The model under review builds one solid part; all positions refer to its coordinate system, in mm. A direction names the side the tool comes from. Coordinates: 2 decimals unless noted, no trailing zeros. Write each loop counter-clockwise with the first axis right and the second up, starting at its lowest first coordinate (ties: lowest second). Pieces come first, ordered by that corner, then holes. Notation, with made-up numbers: (-38.75, 80) - (-11.75, 80) arc R19 cw to (-11.75, 93) - close; hole circle Ø3 at (-34.75, 2.25). An arc over 180 degrees is marked (long way). Put each result on its own line as item: value. Start each with the question number.
Item 1: Consider section D-D on y = -10.5. Give the boundary of the cut face in (x, z), then the cut area to 3 significant figures.
Item 2: Consider section B-B on z = -35. Give the boundary of the cut face in (x, y).
Item 3: Consider section A-A on x = -32.5. Give the boundary of the cut face in (y, z).
Item 4: Consider section C-C on y = 0. State how many separate pieces and enclosed holes the cut face has, then the cut area to 3 significant figures.
Item 5: For pin 1 (6 mm diameter, centred on x = -101.5, y = -4.5, fed in from +Z); pin 2 (15.5 mm diameter, centred on y = -4, z = -22.5, fed in from +X); pin 3 (5 mm diameter, centred on x = -105, y = 0, fed in from -Z); pin 4 (2 mm diameter, centred on x = 0, y = -12, fed in from -Z), all flat-tipped, find the tip position at first contact; note any pin that passes through.
Item 6: Mouldability with a two-part tool opening along X and no side actions: class faces 4 (the face through (-93, 0, -23)), 5 (the face through (95, 0, -23)), 6 (the face through (-95, 0, -22)), 7 (the face through (-107, -4, -38)) as pulls with the +X half, pulls with the -X half, needs draft (parallel to the pull), parting line crosses it, or undercut.
Item 7: To check wall thickness, follow L1, parallel to X at y = 13, z = -18.5; L2, parallel to Z at x = -102.5, y = 13.5; L3, parallel to Y at x = 32, z = -6. State the ranges of each line that lie inside material, in increasing order. Write a range as [from, to].
Item 8: Machinability: for faces 1 (the face through (-1, 0, -7)), 2 (the face through (107, -4, -38)), 3 (the face through (-107, -4, -40)), which of the approach directions +Z, -Z, +X, -X, +Y, -Y give a long, thin tool a straight path to every point of the face, cutting with its end or side? Answer none if there is none.
```python
from build123d import *

# Parameters (mm, degrees)
F1_DEPTH = 17.5
F2_R     = 4
F3_DEPTH = 25
F4_R     = 4.4
F5_DEPTH = 25
F6_R     = 2


# Not quite as in the source:
# - a feature names something its author has since deleted; it is built from what else it names


with BuildPart() as f1:
    # F0 (on Front) → F1 (new body, symmetric)
    with BuildSketch(Plane.XZ):
        Polygon((95, -38), (95, -5), (-95, -5), (-95, -38), (-115, -38), (-115, -40), (-93, -40), (-93, -7), (93, -7), (93, -40), (115, -40), (115, -38), align=None)
    extrude(amount=F1_DEPTH, both=True)

    # F2 (on face) → F3 (cut)
    with BuildSketch(Plane.XY.offset(-38)):
        with Locations((-105, 0)):
            Circle(F2_R)
        with Locations((105, 0)):
            Circle(F2_R)
    extrude(amount=-F3_DEPTH, mode=Mode.SUBTRACT)

    # F4 (on face) → F5 (cut)
    with BuildSketch(Plane.XY.offset(-5)):
        with Locations((-32.5, 0)):
            Circle(F4_R)
        with Locations((32.5, 0)):
            Circle(F4_R)
    extrude(amount=-F5_DEPTH, mode=Mode.SUBTRACT)

    # F6
    f6_edges = [f1.edges().sort_by_distance(p)[0] for p in [
        (95, 0, -5),
        (-95, 0, -5),
        (-93, 0, -40),
        (93, 0, -40),
    ]]
    fillet(f6_edges, radius=F6_R)


solid = f1.part
```
Report:
1. outline: (-115, -40) - (-95, -40) arc R2 ccw to (-93, -38) - (-93, -7) - (93, -7) - (93, -38) arc R2 ccw to (95, -40) - (115, -40) - (115, -38) - (95, -38) - (95, -7) arc R2 ccw to (93, -5) - (-93, -5) arc R2 ccw to (-95, -7) - (-95, -38) - (-115, -38) - close
1. area: 589 mm²
2. outline: (-95, -17.5) - (-93, -17.5) - (-93, 17.5) - (-95, 17.5) - close; (93, -17.5) - (95, -17.5) - (95, 17.5) - (93, 17.5) - close
3. outline: (-17.5, -7) - (-4.4, -7) - (-4.4, -5) - (-17.5, -5) - close; (4.4, -7) - (17.5, -7) - (17.5, -5) - (4.4, -5) - close
4. separate pieces: 5
4. enclosed holes: 0
4. area: 521 mm²
5. pin 1: z = -38
5. pin 2: x = 95
5. pin 3: through
5. pin 4: z = -7
6. face 4: undercut
6. face 5: pulls with the +X half
6. face 6: pulls with the -X half
6. face 7: needs draft
7. L1: [-95, -93], [93, 95]
7. L2: [-40, -38]
7. L3: [-17.5, -4.37], [4.37, 17.5]
8. face 1: -Z, +Y, -Y
8. face 2: +Z, +X, +Y, -Y
8. face 3: -Z, +X, -X, +Y, -Y
